```python
from build123d import *

# Parameters (mm, degrees)
F4_R = 5.99999


# Not quite as in the source:
# - a fillet or chamfer is up to 0.001 mm smaller than in the source, because OpenCascade refuses the exact size


with BuildPart() as f1:
    # F0 (on Front) → F1 (revolve)
    with BuildSketch(Plane.XZ):
        with BuildLine():
            Line((0, 31), (0, 0))
            Line((0, 0), (88, 0))
            Line((88, 0), (88, 16))
            Line((88, 16), (85, 16))
            Line((85, 16), (85, 20))
            Line((85, 20), (68, 20))
            Line((68, 20), (68, 31))
            Line((68, 31), (56, 31))
            ThreePointArc((56, 31), (50, 25), (44, 31))
            Line((44, 31), (0, 31))
        make_face()
    revolve(axis=Axis((68.2048197045, 0, 0), (1, 0, 0)))

    # F2 (on Front) → F3 (revolve, cut)
    with BuildSketch(Plane.XZ):
        Polygon((1.5, 25), (0, 25), (0, 0), (88, 0), (88, 6), (30, 6), (30, 16), (22, 16), (22, 20.5), (19, 20.5), (19, 12.5), (12, 12.5), (12, 16), (1.5, 16), align=None)
    revolve(axis=Axis((-8.4996176884, 0, 0), (-1, 0, 0)), mode=Mode.SUBTRACT)

    # F4 (radius 6 in the source; OpenCascade refuses exactly that, so slightly less here)
    f4_edges = [f1.edges().sort_by_distance(p)[0] for p in [
        (0, 0, -31),
    ]]
    fillet(f4_edges, radius=F4_R)


solid = f1.part
```
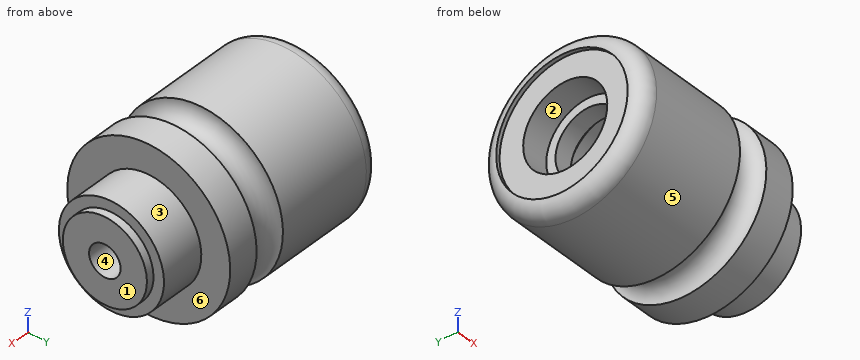
The listing builds one solid part. Answer for the finished solid, in the listing's coordinates (mm). Face numbers are marked on the shaded views. A direction names the side the tool comes from. Coordinates: 2 decimals unless noted, no trailing zeros. Write each loop counter-clockwise with the first axis right and the second up, starting at its lowest first coordinate (ties: lowest second). Pieces come first, ordered by that corner, then holes.
Q1. Which of the six approach directions +Z, -Z, +X, -X, +Y, -Y give full straight-line access (tool end or side, diameter ignored) to the marked faces 1, 2 and 3?
Returned:
face 1: +Z, -Z, +X, +Y, -Y
face 2: -X
face 3: +X
Q2. Find the intervals of material crossed by line 1 along Y through (x, z) = (69, 0); line 2 along Y through (x, z) = (20.45, 0); line 3 along Z through (x, y) = (17.5, -1), in increasing order.
Returned:
line 1: y = -20 to -6, 6 to 20
line 2: y = -31 to -20.5, 20.5 to 31
line 3: z = -30.98 to -12.46, 12.46 to 30.98
Q3. Given P1, Ø9.5, axis at y = 2, z = -7, coming from the -X side; P2, Ø20.5, axis at y = 5, z = 3.5, coming from the -X side; P3, Ø4, axis at x = 22.5, z = 5.5, coming from the -Y side, each flat-ended and moving along its own axis, determine where each tip first touches the part or whether it passes through.
Returned:
P1: stops at x = 30
P2: stops at x = 1.5
P3: stops at y = -30.8
Q4. The mould has two halves that part along Z. Classify the marked faces 4, 5 and 6: released by +Z, released by -Z, zero draft, split by the parting line, or undercut.
Returned:
face 4: undercut
face 5: split by the parting line
face 6: zero draft
Q5. Section A-A, the plane x = 40 is taken. Write down the section's boundary in (y, z).
Returned:
outline: circle Ø62 at (0, 0); hole circle Ø12 at (0, 0)
Q6. Section B-B, the plane x = 9 is taken. Write down the section's boundary in (y, z).
Returned:
outline: circle Ø62 at (0, 0); hole circle Ø32 at (0, 0)
